Geometry check sheet. Reference: drawing and pictorial views, mm from the part's lowest x, y, z. A direction names the side the tool comes from. Round coordinates to 2 decimals unless told otherwise and drop trailing zeros. Order: outer loops, then holes, each group sorted by start corner. A loop starts at its lowest first (then second) coordinate and runs counter-clockwise, first axis right, second up. Notation, with made-up numbers: (2.25, -34.75) -> (57.25, -34.75) arc R6 cw to (57.25, -30.75) -> close; hole circle Ø1 at (84, -14.5). An arc over 180 degrees is marked (long way). Return JSON: item names as keys, results as strings. Group by question number.
1) Section check A-A on x = 14. Enter the section's corners in (y, z), plus the area to 3 significant figures.
2) Draft check along Z on the marked faces 4, 5 and 6. Enter one of: pulls with the +Z half, pulls with the -Z half, needs draft (parallel to the pull), parting line crosses it, or undercut.
3) Section check C-C on x = 8.5. Enter the section's corners in (y, z), plus the area to 3 significant figures.
4) Scan lines: L1, parallel to Z at x = 7.25, y = 32.5; L2, parallel to Z at x = 17, y = 42.5; L3, parallel to X at y = 21.5, z = 15. Record each from-to range of solid material in increasing order.
5) Tool access check on the marked faces 1, 2 and 3. Record the directions out of +Z, -Z, +X, -X, +Y, -Y that give a thin tool (end or side, any length) a straight path to the whole face; none if there is none.
6) Section check B-B on z = 10.5. Enter the section's corners in (x, y) (1 decimal).
7) Section check D-D on y = 12. Enter the section's corners in (x, z).
8) Depth check by flat-ended pin: pin 1 (5 mm diameter, centred on x = 11.5, z = 23, fed in from +Y); pin 2 (0.6 mm diameter, centred on y = 22.5, z = 15, fed in from +X). Enter the tip coordinate at first touch or a pass-through.
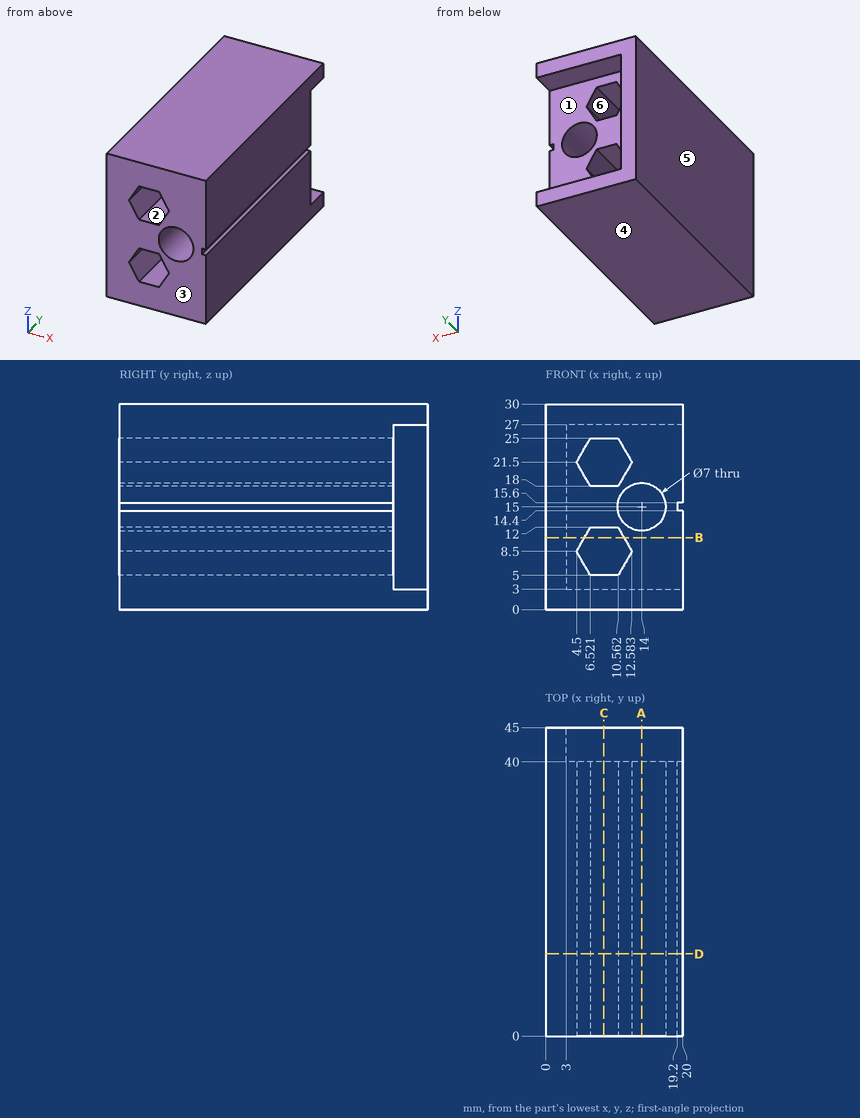
Check result:
{
 "1": {"outline": "(0, 0) -> (45, 0) -> (45, 3) -> (40, 3) -> (40, 11.5) -> (0, 11.5) -> close; (0, 18.5) -> (40, 18.5) -> (40, 27) -> (45, 27) -> (45, 30) -> (0, 30) -> close", "area": "950 mm^2"},
 "2": {"face 4": "pulls with the -Z half", "face 5": "needs draft", "face 6": "undercut"},
 "3": {"outline": "(0, 0) -> (45, 0) -> (45, 3) -> (40, 3) -> (40, 5) -> (0, 5) -> close; (0, 12) -> (40, 12) -> (40, 18) -> (0, 18) -> close; (0, 25) -> (40, 25) -> (40, 27) -> (45, 27) -> (45, 30) -> (0, 30) -> close", "area": "670 mm^2"},
 "4": {"L1": "0 to 5, 12 to 18, 25 to 30", "L2": "0 to 3, 27 to 30", "L3": "0 to 10.5, 17.5 to 19.2"},
 "5": {"face 1": "+X, +Y", "face 2": "+Y, -Y", "face 3": "+Z, -Z, +X, -X, -Y"},
 "6": {"outline": "(0, 0) -> (5.7, 0) -> (5.7, 40) -> (3, 40) -> (3, 45) -> (0, 45) -> close; (11.4, 0) -> (20, 0) -> (20, 40) -> (11.4, 40) -> close"},
 "7": {"outline": "(0, 0) -> (20, 0) -> (20, 14.4) -> (19.2, 14.4) -> (19.2, 15.6) -> (20, 15.6) -> (20, 30) -> (0, 30) -> close; hole (4.5, 8.5) -> (6.52, 5) -> (10.56, 5) -> (12.58, 8.5) -> (10.56, 12) -> (6.52, 12) -> close; hole (4.5, 21.5) -> (6.52, 18) -> (10.56, 18) -> (12.58, 21.5) -> (10.56, 25) -> (6.52, 25) -> close; hole circle Ø7 at (14, 15)"},
 "8": {"pin 1": "y = 40", "pin 2": "x = 19.2"}
}
